Verification items for the finished model (mm, model axes). A direction names the side the tool comes from. Coordinates: 2 decimals unless noted, no trailing zeros. Loops run counter-clockwise (first coordinate to the right, second up) from the corner with the lowest first, then second, coordinate; pieces in that order, holes last.
Q1. Mould release check, pull along Y, two halves, no side actions. Record for faces 6 (the face through (-10.641, -4.563, 17.027)), 7 (the face through (-5, 28.7, 15)), 8 (the face through (-5.417, 6.445, 14.826)): +Y half, -Y half, draft (parallel to the pull), parting line (faces both ways), or undercut.
Q2. Sectioned sample at D-D (x = -12.5). Enter the section's corners in (y, z).
Q3. Go/stop test with flat-tipped pins: P1, Ø12, axis at y = 24, z = 15.5, coming from the -X side; P2, Ø6, axis at x = -12.5, z = 15, coming from the -Y side; P3, Ø5, axis at y = 16, z = 14, coming from the -X side; P4, Ø5, axis at x = -4, z = 19.5, coming from the -Y side. Record where each tip stops, or that it passes through.
Q4. Sectioned sample at C-C (y = -10). Enter the section's corners in (x, z).
Q5. Sectioned sample at B-B (x = -8). Enter the section's corners in (y, z).
Q6. Sectioned sample at A-A (z = 15). Enter the section's corners in (x, y).
Q7. Access from +Z, -Z, +X, -X, +Y, -Y to the whole of each face (thin tool, end or side, straight path). Record for faces 1 (the face through (-8, 0, 15)), 2 (the face through (-5, 15, 1.3)), 3 (the face through (-5.417, 23.555, 14.826)), 4 (the face through (-5, 15, 28.7)), 5 (the face through (-12.28, -12.042, 19.995)).
Q8. Material ranges on probe 1 along X at (y, z) = (-4.5, 15); probe 2 along Y at (x, z) = (-9.5, 2); probe 3 along Y at (x, z) = (-5, 23), recorded low to high.
```python
from build123d import *

# Parameters (mm, degrees)
RESSALTO_EXTRUS_O1_DEPTH = 30
ESBO_O2_R                = 5
CORTE_EXTRUS_O1_DEPTH    = 6
CHANFRO1_SIZE            = 7
ESBO_O3_R                = 2.75
CORTE_EXTRUS_O2_DEPTH    = 54.1130869
ESBO_O4_W                = 27.4
ESBO_O4_H                = 27.4
RESSALTO_EXTRUS_O2_DEPTH = 10
ESBO_O5_W                = 24.8
ESBO_O5_H                = 24.8
CORTE_EXTRUS_O3_DEPTH    = 12
CORTE_EXTRUS_O3_DRAFT    = -40


with BuildPart() as part:
    # Esboço1 → Ressalto-extrusão1 (new body)
    with BuildSketch(Plane.XY):
        Polygon((0, 0), (0, 30), (2, 30), (10, 0), (10, -6), (-6, -15), (-20, -15), (-20, 0), align=None)
    extrude(amount=RESSALTO_EXTRUS_O1_DEPTH)

    # Esboço2 → Corte-extrusão1 (cut)
    with BuildSketch(Plane.XZ.offset(15)):
        with Locations(Location((-12.5, 15, 0), (0, 0, 270))):
            Circle(ESBO_O2_R)
    extrude(amount=-CORTE_EXTRUS_O1_DEPTH, mode=Mode.SUBTRACT)

    # Chanfro1
    chanfro1_edges = [part.edges().sort_by_distance(p)[0] for p in [
        (2, -10.5, 30),
        (10, -3, 30),
    ]]
    chamfer(chanfro1_edges, length=CHANFRO1_SIZE)

    # Esboço3 → Corte-extrusão2 (cut, through all)
    with BuildSketch(Plane.XZ.offset(9)):
        with Locations(Location((-12.5, 15, 0), (0, 0, 270))):
            Circle(ESBO_O3_R)
    extrude(amount=-CORTE_EXTRUS_O2_DEPTH, mode=Mode.SUBTRACT)

    # Esboço4 → Ressalto-extrusão2 (add)
    with BuildSketch(Plane.ZY):
        with Locations((15, 15)):
            Rectangle(ESBO_O4_W, ESBO_O4_H)
    extrude(amount=RESSALTO_EXTRUS_O2_DEPTH)


with BuildPart() as corte_extrus_o3_tool:
    # Esboço5 → Corte-extrusão3 (with draft: the straight prism first)
    with BuildSketch(Plane.ZY.offset(10)):
        with Locations((15, 15)):
            Rectangle(ESBO_O5_W, ESBO_O5_H)
    extrude(amount=-CORTE_EXTRUS_O3_DEPTH)
    # Corte-extrusão3: the draft: its side faces are tilted about the plane it starts from
    corte_extrus_o3_sides = [corte_extrus_o3_tool.faces().sort_by_distance(p)[0] for p in [
        (-4, 27.4, 15),
        (-4, 15, 2.6),
        (-4, 2.6, 15),
        (-4, 15, 27.4),
    ]]
    draft(corte_extrus_o3_sides, Plane.ZY.offset(10), CORTE_EXTRUS_O3_DRAFT)


with BuildPart() as part_1:
    add(part.part)

    # Corte-extrusão3: cut by corte_extrus_o3_tool
    add(corte_extrus_o3_tool.part, mode=Mode.SUBTRACT)


solid = part_1.part
```
Geometry check:
1. face 6: draft
1. face 7: +Y half
1. face 8: undercut
2. outline: (-15, 0) - (0, 0) - (0, 12.25) - (-9, 12.25) - (-9, 10) - (-15, 10) - close; (-15, 20) - (-9, 20) - (-9, 17.75) - (0, 17.75) - (0, 30) - (-10.62, 30) - (-15, 26.19) - close
3. P1: stops at x = -10
3. P2: stops at y = -9
3. P3: stops at x = 0.61
3. P4: stops at y = -15
4. outline: (-20, 0) - (2.89, 0) - (2.89, 23) - (-11.39, 30) - (-20, 30) - close; hole circle Ø10 at (-12.5, 15)
5. outline: (-15, 0) - (0, 0) - (0, 30) - (-8.09, 30) - (-15, 23.98) - (-15, 17.18) - (-9, 17.18) - (-9, 12.82) - (-15, 12.82) - close; (1.3, 1.3) - (28.7, 1.3) - (28.7, 28.7) - (1.3, 28.7) - close; hole (4.28, 4.28) - (25.72, 4.28) - (25.72, 25.72) - (4.28, 25.72) - close
6. outline: (-20, -15) - (-17.5, -15) - (-17.5, -9) - (-15.25, -9) - (-15.25, 0) - (-20, 0) - close; (-10, 1.3) - (0, 1.3) - (0, 0) - (-9.75, 0) - (-9.75, -9) - (-7.5, -9) - (-7.5, -15) - (-6, -15) - (10, -6) - (10, 0) - (2, 30) - (0, 30) - (0, 28.7) - (-10, 28.7) - (-10, 27.4) - (2, 17.33) - (2, 12.67) - (-10, 2.6) - close
7. face 1: +Z, -Z, -X
7. face 2: -Z, -X, +Y
7. face 3: -X
7. face 4: +Z, -X, +Y
7. face 5: -Y
8. probe 1: x = -20 to -15.25, -9.75 to 10
8. probe 2: y = -15 to 0, 1.3 to 28.7
8. probe 3: y = -14.44 to 0, 1.3 to 6.8, 23.2 to 28.7
